CAD build for the part. Positions are in the model's coordinates, mm. Give positions to 0.01 mm unless a question says otherwise; leave off trailing zeros. Order: outer loops, then holes, each group sorted by start corner. A loop starts at its lowest first (then second) coordinate and runs counter-clockwise, first axis right, second up. Notation, with made-up numbers: (-22, -25.75) -> (-9, -25.75) arc R14 cw to (-9, -15.75) -> close; hole circle Ø7 at (-6, -21.75). An arc over 180 degrees is marked (long way). Answer as CSV lines item,"result".
Autodesk Inventor part; units mm, degrees
ref_plane "YZ Plane" through (0, 0, 0) normal (1, 0, 0) x (0, 1, 0)
ref_plane "XZ Plane" through (0, 0, 0) normal (0, 1, 0) x (-1, 0, 0)
ref_plane "XY Plane" through (0, 0, 0) normal (0, 0, 1) x (1, 0, 0)
sketch "Skizze_Grudnkörper" plane through (0, 0, 0) normal (0, 0, 1) x (1, 0, 0)
  circle A0 centre (0, 0) radius 4
  dimension "d0" = 8
extrude "Grundkörper" add sketch "Skizze_Grudnkörper" along normal blind 30
hole "Bohrung_4_mm" at (0, 0, 30) direction (0, 0, -1) diameter 4 depth 10 tip angle 118
sketch "Skizze2" plane through (0, 0, 0) normal (0, 1, 0) x (-1, 0, 0)
  line L0 (-4, 0) -> (-4, 30)
  line L1 (-4, 30) -> (-2, 30)
  line L2 (-2, 30) -> (-2, 20)
  line L3 (-2, 20) -> (0, 18.7983)
  line L4 (0, 18.7983) -> (2, 20)
  line L5 (2, 20) -> (2, 30)
  line L6 (2, 30) -> (4, 30)
  line L7 (4, 30) -> (4, 0)
  line L8 (4, 0) -> (-4, 0)
  line L9 (5.6, 0) -> (-5.6, 0)
  line L10 (0, -6) -> (0, 36)
  circle A0 centre (0, 10) radius 10
  point P0 (0, 0)
  point P1 (4, 0.8348)
  point P2 (0, 0)
  dimension "d12" = 20
revolve "Kugel" cut sketch "Skizze2" angle 360 about axis through (0, 0, -10) along (0, 0, 1) contours A0 L7 L8
properties material "Stahl, Legierung"
1) Pin check, flat tips, straight feed: P1, Ø3, axis at x = -3, y = 0, coming from the -Z side; P2, Ø3, axis at y = 3, z = 25, coming from the -X side; P3, Ø4, axis at y = 3, z = 20.5, coming from the -X side. Stop position of each tip, or through.
Data:
P1,"stops at z = 0.11"
P2,"stops at x = -3.71"
P3,"stops at x = -3.87"
2) Band-saw the part on B-B, the plane z = 6.5. Write the cut outline in (x, y), then the cut area to 3 significant figures.
Data:
outline,"circle Ø8 at (0, 0)"
area,"50.3 mm2"
3) Band-saw the part on D-D, the plane y = 2.5. Write the cut outline in (x, z), then the cut area to 3 significant figures.
Data:
outline,"(-3.12, 0.83) arc R9.68 ccw to (3.12, 0.83) -> (3.12, 30) -> (-3.12, 30) -> close"
area,"184 mm2"
4) Pull direction X, two halves, no side cores. Call faces 1 (the cylindrical face through (2, 0, 25)), 2 (the flat face through (-2, -1, 30)), 3 (the cylindrical face through (-0.867, 3.905, 15.213)): pulls with the +X half, pulls with the -X half, needs draft (parallel to the pull), parting line crosses it, or undercut.
Data:
face 1,"undercut"
face 2,"needs draft"
face 3,"parting line crosses it"
5) Wall check: line 1 along X through (y, z) = (0, 24.5); line 2 along Y through (x, z) = (-1.5, 20.5). Give the ranges that are in metal, low to high. Write a range as [from, to].
Data:
line 1,"x = [-4, -2], [2, 4]"
line 2,"y = [-3.71, -1.32], [1.32, 3.71]"
6) Band-saw the part on C-C, the plane x = -3. Write the cut outline in (y, z), then the cut area to 3 significant figures.
Data:
outline,"(-2.65, 0.83) arc R9.54 ccw to (2.65, 0.83) -> (2.65, 30) -> (-2.65, 30) -> close"
area,"156 mm2"
7) Band-saw the part on A-A, the plane z = 27.5. Write the cut outline in (x, y).
Data:
outline,"circle Ø8 at (0, 0); hole circle Ø4 at (0, 0)"
